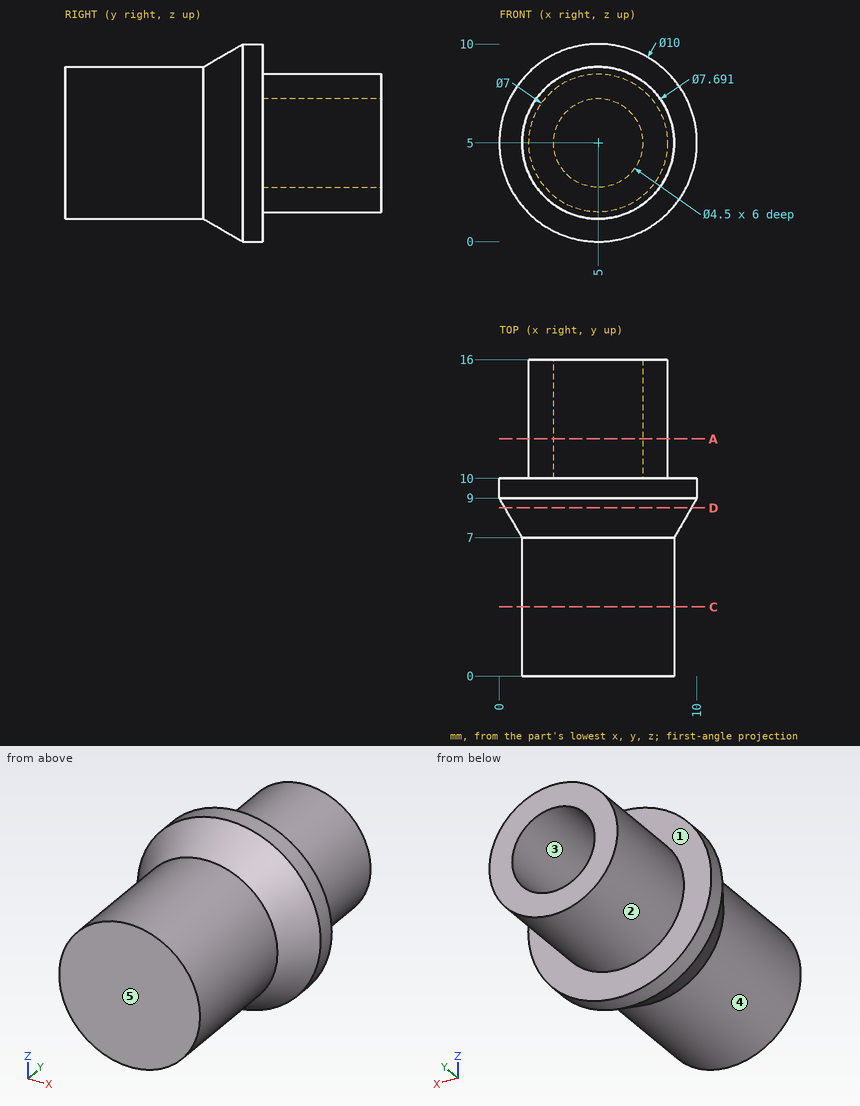
Here's the drawing with two shaded views (mm, measured from the low corner). I have some questions. A direction names the side the tool comes from. Give positions to 0.01 mm unless a question says otherwise; leave off trailing zeros. Loops run counter-clockwise (first coordinate to the right, second up) from the corner with the lowest first, then second, coordinate; pieces in that order, holes last. Notation, with made-up numbers: M 21.5,-13 L 34.5,-13 A16 cw 34.5,5 Z; hole C 27,-34.5 d2. An arc over 180 degrees is marked long. One line per item, written item: value.
(1) Will these pins go through, and if not, where does the flat tip stop? pin 1 (2 mm diameter, centred on x = 5.5, z = 5, fed in from +Y); pin 2 (3 mm diameter, centred on x = 7, y = 6.5, fed in from -Z); pin 3 (5 mm diameter, centred on x = 6.5, y = 6, fed in from +Z) (1 decimal).
Returned:
pin 1: y = 10
pin 2: z = 0.88
pin 3: z = 9.6
(2) Suppose I cut it at A-A on y = 12. List the corners of the cut face in (x, z) for me, plus the area to 3 significant figures.
Returned:
outline: C 5,5 d7; hole C 5,5 d4.5
area: 22.6 mm^2
(3) We'd pull the mould along Z, two halves only. Please class the marked faces 1, 2 and 3: released by +Z, released by -Z, zero draft, split by the parting line, or undercut.
Returned:
face 1: zero draft
face 2: split by the parting line
face 3: undercut
(4) Suppose I cut it at D-D on y = 8.5. List the corners of the cut face in (x, z) for me.
Returned:
outline: C 5,5 d9.42
(5) Which directions (+Z, -Z, +X, -X, +Y, -Y) give clear straight access to the entire face, cutting with the end or side of a thin tool? Please do the marked faces 4 and 5.
Returned:
face 4: -Y
face 5: +Z, -Z, +X, -X, -Y
(6) I need wall thicknesses on line 1 (Z direction, x = 5, y = 11.3); line 2 (Y direction, x = 3.75, z = 8.5); line 3 (X direction, y = 14.5, z = 3.25) (1 decimal). Which ranges of each line are inside material? Lowest first, please.
Returned:
line 1: 1.5 to 2.75, 7.25 to 8.5
line 2: 0 to 10
line 3: 2 to 3.6, 6.4 to 8
(7) Suppose I cut it at C-C on y = 3.5. List the corners of the cut face in (x, z) for me (1 decimal).
Returned:
outline: C 5,5 d7.7
